Read the model definition and answer for the solid it produces. Units are mm, in the model's axes. A direction names the side the tool comes from. Give positions to 0.01 mm unless a question says otherwise; leave off trailing zeros. Write each loop counter-clockwise with the first axis right and the second up, starting at its lowest first coordinate (ties: lowest second). Pieces come first, ordered by that corner, then holes.
```python
from build123d import *


with BuildPart() as f1:
    # F0 (on Front) → F1 (revolve)
    with BuildSketch(Plane.XZ):
        with BuildLine():
            Line((0, 31), (0, 0))
            Line((0, 0), (88, 0))
            Line((88, 0), (88, 15))
            Line((88, 15), (85, 15))
            Line((85, 15), (85, 20))
            Line((85, 20), (68, 20))
            Line((68, 20), (68, 31))
            Line((68, 31), (56, 31))
            ThreePointArc((56, 31), (50, 25), (44, 31))
            Line((44, 31), (0, 31))
        make_face()
    revolve(axis=Axis((113.79065, 0, 0), (1, 0, 0)))

    # F2 (on Front) → F3 (revolve, cut)
    with BuildSketch(Plane.XZ):
        Polygon((0, 25), (0, 0), (93, 0), (93, 6), (23, 6), (23, 20.5), (15, 20.5), (15, 12.5), (12, 12.5), (12, 16), (1.5, 16), (1.5, 25), align=None)
    revolve(axis=Axis((46.5, 0, 0), (-1, 0, 0)), mode=Mode.SUBTRACT)


solid = f1.part
```
Item 1: Section A-A (x = 69.5) is taken. Write down the section's boundary in (y, z).
Result set:
outline: circle Ø40 at (0, 0); hole circle Ø12 at (0, 0)
Item 2: Each of these flat-tipped pins is pushed along its axis until it touches: pin 1 Ø1 at (x, y) = (12.5, -18) entering from +Z; pin 2 Ø3 at (y, z) = (8.5, -1) entering from -X; pin 3 Ø4 at (y, z) = (11.5, 11) entering from -X. Where does it stop, or does it pass through?
Result set:
pin 1: stops at z = 25.59
pin 2: stops at x = 23
pin 3: stops at x = 1.5
Item 3: Which of the six approach directions +Z, -Z, +X, -X, +Y, -Y give full straight-line access (tool end or side, diameter ignored) to faces 1 (the flat face through (23, 5, -4)), 2 (the flat face through (85, -15, -3)), 3 (the flat face through (1.5, -16.3, 0.3))?
Result set:
face 1: none
face 2: +X
face 3: -X
Item 4: Find the intervals of material crossed by line 1 along Y through (x, z) = (14, 0); line 2 along Y through (x, z) = (7.75, 0); line 3 along X through (y, z) = (10, -17), in increasing order.
Result set:
line 1: y = -31 to -12.5, 12.5 to 31
line 2: y = -31 to -16, 16 to 31
line 3: x = 1.5 to 15, 23 to 85
Item 5: Section B-B (x = 17) is taken. Write down the section's boundary in (y, z).
Result set:
outline: circle Ø62 at (0, 0); hole circle Ø41 at (0, 0)
Item 6: Determine the mould class of faces 4 (the cylindrical face through (86.479, -0.66, -14.985)), 5 (the flat face through (15, -9, -9)), 6 (the flat face through (68, 20.2, 0.4)) for opening direction X: pulls with the +X half, pulls with the -X half, needs draft (parallel to the pull), parting line crosses it, or undercut.
Result set:
face 4: needs draft
face 5: undercut
face 6: pulls with the +X half
